```python
from build123d import *

# Parameters (mm, degrees)
SKETCH1_W           = 140
SKETCH1_H           = 140
BOSS_EXTRUDE1_DEPTH = 2
BOSS_EXTRUDE3_DEPTH = 2
SKETCH3_R           = 2
CUT_EXTRUDE1_DEPTH  = 2
FILLET1_R           = 10
SKETCH4_R           = 1.5
CUT_EXTRUDE2_DEPTH  = 2
CUT_EXTRUDE3_DEPTH  = 2


with BuildPart() as part:
    # Sketch1 → Boss-Extrude1 (new body)
    with BuildSketch(Plane(origin=(0, 0, 0), x_dir=(1, 0, 0), z_dir=(0, 1, 0))):
        with Locations((70, 70)):
            Rectangle(SKETCH1_W, SKETCH1_H)
    extrude(amount=BOSS_EXTRUDE1_DEPTH)

    # Sketch2 → Boss-Extrude3 (add)
    with BuildSketch(Plane(origin=(0, 2, 0), x_dir=(1, 0, 0), z_dir=(0, 1, 0))):
        Polygon((111.715728753, 140), (140, 111.715728753), (154.142135624, 125.857864376), (125.857864376, 154.142135624), align=None)
        Polygon((0, 111.715728753), (-14.142135624, 125.857864376), (14.142135624, 154.142135624), (28.284271247, 140), align=None)
        Polygon((28.284271247, 0), (0, 28.284271247), (-14.142135624, 14.142135624), (14.142135624, -14.142135624), align=None)
        Polygon((140, 28.284271247), (154.142135624, 14.142135624), (125.857864376, -14.142135624), (111.715728753, 0), align=None)
    extrude(amount=-BOSS_EXTRUDE3_DEPTH)

    # Sketch3 → Cut-Extrude1 (cut)
    with BuildSketch(Plane(origin=(0, 2, 0), x_dir=(1, 0, 0), z_dir=(0, 1, 0))):
        with Locations(Location((7.07813888, 0.360624458, 0), (0, 0, 270))):
            Circle(SKETCH3_R)
        with Locations(Location((0.360624458, 7.07813888, 0), (0, 0, 90))):
            Circle(SKETCH3_R)
        with Locations(Location((41.372817767, 34.655303346, 0), (0, 0, 90))):
            Circle(SKETCH3_R)
        with Locations(Location((34.655303346, 41.372817767, 0), (0, 0, 270))):
            Circle(SKETCH3_R)
        with Locations(Location((132.92186112, 0.360624458, 0), (0, 0, 90))):
            Circle(SKETCH3_R)
        with Locations(Location((139.639375542, 7.07813888, 0), (0, 0, 270))):
            Circle(SKETCH3_R)
        with Locations(Location((98.627182233, 34.655303346, 0), (0, 0, 270))):
            Circle(SKETCH3_R)
        with Locations(Location((105.344696654, 41.372817767, 0), (0, 0, 90))):
            Circle(SKETCH3_R)
        with Locations(Location((132.92186112, 139.639375542, 0), (0, 0, 270))):
            Circle(SKETCH3_R)
        with Locations(Location((139.639375542, 132.92186112, 0), (0, 0, 90))):
            Circle(SKETCH3_R)
        with Locations(Location((98.627182233, 105.344696654, 0), (0, 0, 90))):
            Circle(SKETCH3_R)
        with Locations(Location((105.344696654, 98.627182233, 0), (0, 0, 270))):
            Circle(SKETCH3_R)
        with Locations(Location((7.07813888, 139.639375542, 0), (0, 0, 90))):
            Circle(SKETCH3_R)
        with Locations(Location((0.360624458, 132.92186112, 0), (0, 0, 270))):
            Circle(SKETCH3_R)
        with Locations(Location((41.372817767, 105.344696654, 0), (0, 0, 270))):
            Circle(SKETCH3_R)
        with Locations(Location((34.655303346, 98.627182233, 0), (0, 0, 90))):
            Circle(SKETCH3_R)
        Polygon((13.795653301, -0.346482323), (42.079924548, 27.937788925), (27.937788925, 42.079924548), (-0.346482323, 13.795653301), align=None)
        Polygon((97.920075452, 27.937788925), (112.062211075, 42.079924548), (140.346482323, 13.795653301), (126.204346699, -0.346482323), align=None)
        Polygon((126.204346699, 140.346482323), (97.920075452, 112.062211075), (112.062211075, 97.920075452), (140.346482323, 126.204346699), align=None)
        Polygon((42.079924548, 112.062211075), (27.937788925, 97.920075452), (-0.346482323, 126.204346699), (13.795653301, 140.346482323), align=None)
    extrude(amount=-CUT_EXTRUDE1_DEPTH, mode=Mode.SUBTRACT)

    # Fillet1
    fillet1_edges = [part.edges().sort_by_distance(p)[0] for p in [
        (125.857864376, 1, -154.142135624),
        (154.142135624, 1, -125.857864376),
        (-14.142135624, 1, -125.857864376),
        (14.142135624, 1, -154.142135624),
        (14.142135624, 1, 14.142135624),
        (-14.142135624, 1, -14.142135624),
        (154.142135624, 1, -14.142135624),
        (125.857864376, 1, 14.142135624),
    ]]
    fillet(fillet1_edges, radius=FILLET1_R)

    # Sketch4 → Cut-Extrude2 (cut)
    with BuildSketch(Plane(origin=(0, 2, 0), x_dir=(1, 0, 0), z_dir=(0, 1, 0))):
        with Locations(Location((38.717631804, 10.433360556, 0), (0, 0, 270))):
            Circle(SKETCH4_R)
        with Locations(Location((10.433360556, 38.717631804, 0), (0, 0, 90))):
            Circle(SKETCH4_R)
        with Locations(Location((101.282368196, 10.433360556, 0), (0, 0, 90))):
            Circle(SKETCH4_R)
        with Locations(Location((129.566639444, 38.717631804, 0), (0, 0, 270))):
            Circle(SKETCH4_R)
        with Locations(Location((38.717631804, 129.566639444, 0), (0, 0, 90))):
            Circle(SKETCH4_R)
        with Locations(Location((10.433360556, 101.282368196, 0), (0, 0, 270))):
            Circle(SKETCH4_R)
        with Locations(Location((101.282368196, 129.566639444, 0), (0, 0, 270))):
            Circle(SKETCH4_R)
        with Locations(Location((129.566639444, 101.282368196, 0), (0, 0, 90))):
            Circle(SKETCH4_R)
    extrude(amount=-CUT_EXTRUDE2_DEPTH, mode=Mode.SUBTRACT)

    # Sketch5 → Cut-Extrude3 (cut)
    with BuildSketch(Plane(origin=(0, 2, 0), x_dir=(1, 0, 0), z_dir=(0, 1, 0))):
        Polygon((75, 15), (70, 10), (65, 15), (70, 5), align=None)
    extrude(amount=-CUT_EXTRUDE3_DEPTH, mode=Mode.SUBTRACT)


solid = part.part
```
Source: CAD feature listing. Evaluate the final solid. Frame: model axes, mm. A direction names the side the tool comes from. Round coordinates to 2 decimals unless told otherwise and drop trailing zeros. Loops run counter-clockwise (first coordinate to the right, second up) from the corner with the lowest first, then second, coordinate; pieces in that order, holes last.
(1) Access query for faces 1 (the flat face through (143.486, 1.014, -24.798)), 2 (the flat face through (112.26, 1.01, -13.6)), 3 (the flat face through (24.699, 1.014, -143.585)). Directions: +Z, -Z, +X, -X, +Y, -Y. A direction counts if a zero-diameter tool reaches every point of the face in a straight line with its end or side. Return the directions, or none.
From the geometry:
face 1: +X, +Y, -Y
face 2: +Y, -Y
face 3: -Z, +Y, -Y
(2) Contact query for flat-ended pins moving along their axis: pin 1 Ø0.6 at (y, z) = (1, -89.5) entering from +X; pin 2 Ø1 at (y, z) = (1, -62) entering from -X. Output: stop coordinate, or through.
From the geometry:
pin 1: stops at x = 140
pin 2: stops at x = 0
(3) Section query B-B (z = -24). Output: boundary loops of the cut face in (x, y).
From the geometry:
outline: (-4.28, 0) - (9.86, 0) - (9.86, 2) - (-4.28, 2) - close; (38.14, 0) - (101.86, 0) - (101.86, 2) - (38.14, 2) - close; (130.14, 0) - (144.28, 0) - (144.28, 2) - (130.14, 2) - close
(4) Section query A-A (x = 72). Output: boundary loops of the cut face in (y, z), and give its area (3 significant figures).
From the geometry:
outline: (0, -140) - (2, -140) - (2, -12) - (0, -12) - close; (0, -9) - (2, -9) - (2, 0) - (0, 0) - close
area: 274 mm2
(5) Section query D-D (x = 88.5). Output: boundary loops of the cut face in (y, z), and give its area (3 significant figures).
From the geometry:
outline: (0, -140) - (2, -140) - (2, 0) - (0, 0) - close
area: 280 mm2
(6) Material intervals for probe 1 along Z at (x, y) = (118, 0.3); probe 2 along Z at (x, y) = (19, 1.7); probe 3 along X at (y, z) = (1.2, -6), sorted ascending.
From the geometry:
probe 1: z = -146.28 to -132.14, -103.86 to -36.14, -7.86 to 6.28
probe 2: z = -148.74 to -135.14, -106.86 to -33.14, -4.86 to 8.74
probe 3: x = -6 to -1.32, 2.05 to 7.45, 20.14 to 69.5, 70.5 to 119.86, 132.55 to 137.95, 141.32 to 146
(7) Section query C-C (y = 1.55). Give the number of separate pieces and of enclosed holes in the cut face, and give its area (3 significant figures).
From the geometry:
separate pieces: 1
enclosed holes: 29
area: 17,500 mm2
(8) Pull-direction query (Z, two-part tool) for faces 4 (the flat face through (0, 1, -140)), 5 (the flat face through (69, 2, -71)), 6 (the cylindrical face through (130.94, 1.01, -0.1)); classes: +Z half, -Z half, draft (parallel to the pull), parting line (faces both ways), or undercut.
From the geometry:
face 4: -Z half
face 5: draft
face 6: undercut
